Answer from the drawing. Dimensions are ordinates in mm from the lowest x, y and z of the part. A direction names the side the tool comes from. Coordinates: 2 decimals unless noted, no trailing zeros. Order: outer loops, then holes, each group sorted by start corner. A loop starts at its lowest first (then second) coordinate and runs counter-clockwise, first axis right, second up.
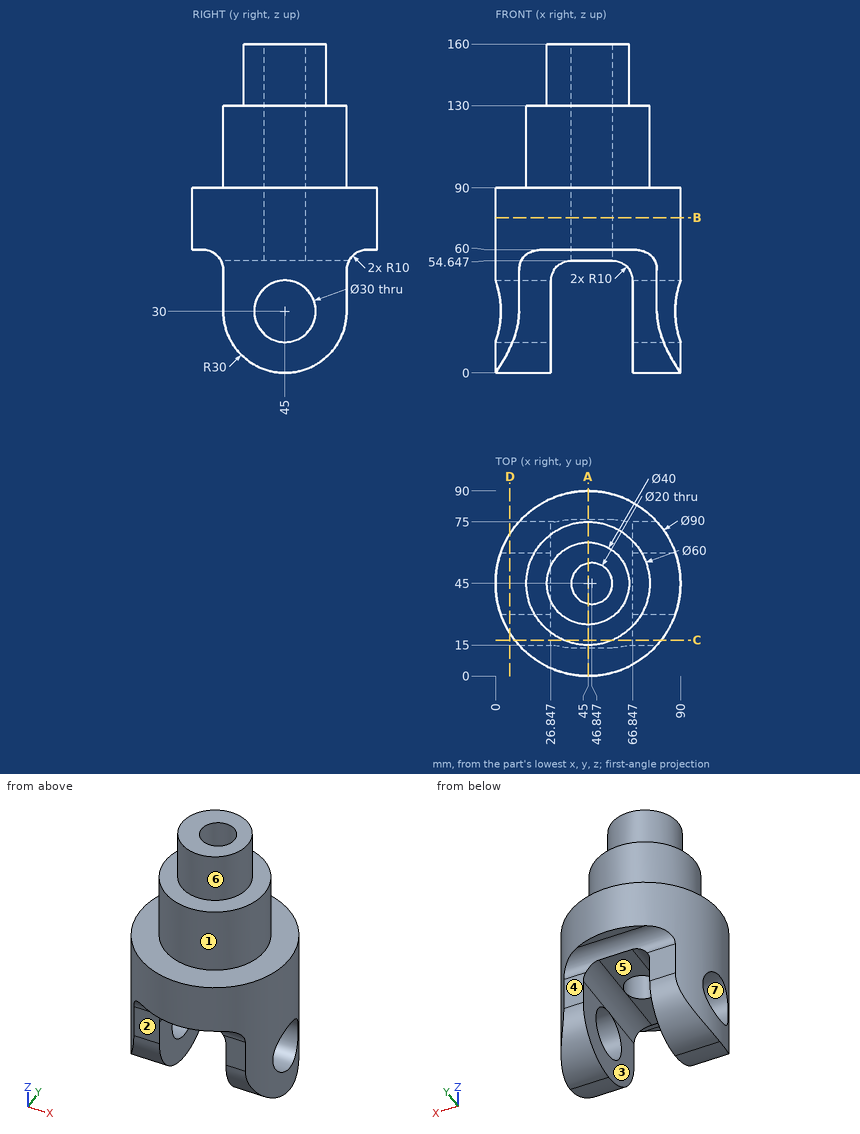
1) Consider L1, parallel to Z at x = 37, y = 65; L2, parallel to Z at x = 38, y = 52; L3, parallel to Z at x = 7, y = 34. Determine where each line is inside the solid, lowest interval first.
2) Determine the mould class of the marked faces 4, 5, 6 and 7 for opening direction Y: released by +Y, released by -Y, zero draft, split by the parting line, or undercut.
3) Section B-B (z = 75.5) is taken. Give the vertices of the cut face in (x, y).
4) A tool of negligible diameter and unlimited length cuts with its end or side. For the marked faces 1, 2 and 3, from which of +Z, -Z, +X, -X, +Y, -Y can it reach the whole face along a straight path? Write none if from no direction.
5) Section D-D (x = 7) is taken. Give the vertices of the cut face in (y, z).
6) Each of these flat-tipped pins is pushed along its axis until it touches: P1, Ø6, axis at x = 12, y = 26, coming from the +Z side; P2, Ø5, axis at y = 19, z = 60, coming from the -X side; P3, Ø12, axis at y = 12.5, z = 71.5, coming from the -X side; P4, Ø12, axis at x = 68.5, y = 36.5, coming from the +Z side. Where does it stop, or does it pass through?
7) Section A-A (x = 45) is taken. Give the vertices of the cut face in (y, z).
8) Section C-C (y = 17.5) is taken. Give the vertices of the cut face in (x, z), then the cut area to 4 significant figures.
Filled sheet:
1. L1: z = 54.65 to 130
1. L2: z = 54.65 to 160
1. L3: z = 2.09 to 19.8, 40.2 to 90
2. face 4: released by +Y
2. face 5: zero draft
2. face 6: split by the parting line
2. face 7: undercut
3. outline: circle Ø90 at (45, 45); hole circle Ø20 at (46.85, 45)
4. face 1: +Z
4. face 2: -Z, +X, -X, -Y
4. face 3: -Z, +Y, -Y
5. outline: (20.9, 12.14) arc R30 ccw to (69.1, 12.14) - (69.1, 90) - (20.9, 90) - close; hole circle Ø30 at (45, 30)
6. P1: stops at z = 90
6. P2: stops at x = 6.62
6. P3: stops at x = 8.63
6. P4: stops at z = 160
7. outline: (0, 60) - (5, 60) arc R10 cw to (13.85, 54.65) - (35.17, 54.65) - (35.17, 160) - (25, 160) - (25, 130) - (15, 130) - (15, 90) - (0, 90) - close; (54.83, 54.65) - (76.15, 54.65) arc R10 cw to (85, 60) - (90, 60) - (90, 90) - (75, 90) - (75, 130) - (65, 130) - (65, 160) - (54.83, 160) - close
8. outline: (9.38, 18.01) - (26.85, 18.01) - (26.85, 44.65) arc R10 cw to (36.85, 54.65) - (56.85, 54.65) arc R10 cw to (66.85, 44.65) - (66.85, 18.01) - (80.62, 18.01) - (80.62, 90) - (56.99, 90) - (56.99, 130) - (33.01, 130) - (33.01, 90) - (9.38, 90) - close
8. area: 4,665 mm2
